```python
from build123d import *

# Parameters (mm, degrees)
CUT_EXTRUDE_1_DEPTH           = 1.2
CUT_EXTRUDE_1_DRAFT           = -30
SKETCH_3_W                    = 3
SKETCH_3_H                    = 12
CUT_EXTRUDE_1_PROFILE_2_DEPTH = 1.2
CUT_EXTRUDE_1_PROFILE_2_DRAFT = -30


with BuildPart() as part:
    # Эскиз1 → Повернуть1 (revolve)
    with BuildSketch(Plane.XY, mode=Mode.PRIVATE) as revolve_1_sk:
        with BuildLine():
            Line((0, 64.100995099), (-26.732050808, 64.100995099))
            Line((-26.732050808, 64.100995099), (-30.196152423, 58.100995099))
            Line((-30.196152423, 58.100995099), (-26.732050808, 58.100995099))
            Line((-26.732050808, 58.100995099), (-25, 61.100995099))
            Line((-25, 61.100995099), (-20, 61.100995099))
            Line((-20, 61.100995099), (-20, 42.100995099))
            Line((-20, 42.100995099), (-19, 41.100995099))
            Line((-19, 41.100995099), (-18, 41.100995099))
            Line((-18, 41.100995099), (-18, 58.100995099))
            ThreePointArc((-18, 58.100995099), (-17.121320344, 60.222315442), (-15, 61.100995099))
            Line((-15, 61.100995099), (0, 61.100995099))
            Line((0, 61.100995099), (0, 64.100995099))
        make_face()
    revolve(revolve_1_sk.sketch.rotate(Axis((0, 61.100995099, 0), (0, 1, 0)), 270), axis=Axis((0, 61.100995099, 0), (0, 1, 0)))


with BuildPart() as cut_extrude_1_tool:
    # Эскиз3 → Вырез-Вытянуть1 (with draft: the straight prism first)
    with BuildSketch(Plane(origin=(0, 64.100995099, 0), x_dir=(1, 0, 0), z_dir=(0, 1, 0))):
        with BuildLine():
            Line((-4.5, 12.196310918), (-4.5, 8.93028555))
            ThreePointArc((-4.5, 8.93028555), (0, -10), (4.5, 8.93028555))
            Line((4.5, 8.93028555), (4.5, 12.196310918))
            ThreePointArc((4.5, 12.196310918), (0, -13), (-4.5, 12.196310918))
        make_face()
    extrude(amount=-CUT_EXTRUDE_1_DEPTH)
    # Вырез-Вытянуть1: the draft: its side faces are tilted about the plane it starts from
    cut_extrude_1_sides = [cut_extrude_1_tool.faces().sort_by_distance(p)[0] for p in [
        (-4.5, 63.500995099, -10.563298234),
        (0, 63.500995099, 10),
        (4.5, 63.500995099, -10.563298234),
        (0, 63.500995099, 13),
    ]]
    draft(cut_extrude_1_sides, Plane(origin=(0, 64.100995099, 0), x_dir=(1, 0, 0), z_dir=(0, 1, 0)), CUT_EXTRUDE_1_DRAFT)


with BuildPart() as part_1:
    add(part.part)

    # Вырез-Вытянуть1: cut by cut_extrude_1_tool
    add(cut_extrude_1_tool.part, mode=Mode.SUBTRACT)


with BuildPart() as cut_extrude_1_profile_2_tool:
    # Эскиз3 → Вырез-Вытянуть1 profile 2 (with draft: the straight prism first)
    with BuildSketch(Plane(origin=(0, 64.100995099, 0), x_dir=(1, 0, 0), z_dir=(0, 1, 0))):
        with Locations((0, 11.509630879)):
            Rectangle(SKETCH_3_W, SKETCH_3_H)
    extrude(amount=-CUT_EXTRUDE_1_PROFILE_2_DEPTH)
    # Вырез-Вытянуть1 profile 2: the draft: its side faces are tilted about the plane it starts from
    cut_extrude_1_profile_2_sides = [cut_extrude_1_profile_2_tool.faces().sort_by_distance(p)[0] for p in [
        (-1.5, 63.500995099, -11.509630879),
        (0, 63.500995099, -5.509630879),
        (1.5, 63.500995099, -11.509630879),
        (0, 63.500995099, -17.509630879),
    ]]
    draft(cut_extrude_1_profile_2_sides, Plane(origin=(0, 64.100995099, 0), x_dir=(1, 0, 0), z_dir=(0, 1, 0)), CUT_EXTRUDE_1_PROFILE_2_DRAFT)


with BuildPart() as part_2:
    add(part_1.part)

    # Вырез-Вытянуть1 profile 2: cut by cut_extrude_1_profile_2_tool
    add(cut_extrude_1_profile_2_tool.part, mode=Mode.SUBTRACT)


solid = part_2.part
```
The model under review builds one solid part; all positions refer to its coordinate system, in mm. A direction names the side the tool comes from. Round coordinates to 2 decimals unless told otherwise and drop trailing zeros. Write each loop counter-clockwise with the first axis right and the second up, starting at its lowest first coordinate (ties: lowest second). Pieces come first, ordered by that corner, then holes. Notation, with made-up numbers: (-2, 38.5) - (8, 38.5) arc R18 ccw to (8, 48.5) - close; hole circle Ø6 at (47, 7.25). An arc over 180 degrees is marked (long way). One line per question, with ' | ' between items.
Item 1: For faces 5 (the face through (17, 41.101, -7)), 6 (the face through (-1, 62.901, 11)), 7 (the face through (-17, 61.101, 11)), list the 3-axis set-ups (+Z, -Z, +X, -X, +Y, -Y) from which the entire face can be reached by the end or side of a thin tool; tool diameter is ignored.
Resolved:
face 5: +Z, -Z, +X, -X, -Y | face 6: +Y | face 7: -Y
Item 2: The part is to be moulded in two halves that separate along Z. For faces 1 (the face through (0, 62.901, -12)), 2 (the face through (24.488, 60.955, 5.438)), 3 (the face through (26.308, 63.726, 5.842)), 4 (the face through (0, 64.101, 0)), say which applies: pulls with the +Z half, pulls with the -Z half, needs draft (parallel to the pull), parting line crosses it, or undercut.
Resolved:
face 1: undercut | face 2: undercut | face 3: parting line crosses it | face 4: needs draft
Item 3: Add section B-B, the plane x = 0. Give the boundary of the cut face in (y, z).
Resolved:
outline: (41.1, -19) - (42.1, -20) - (61.1, -20) - (61.1, -25) - (58.1, -26.73) - (58.1, -30.2) - (64.1, -26.73) - (64.1, -17.51) - (62.9, -16.82) - (62.9, -6.2) - (64.1, -5.51) - (64.1, 10) - (62.9, 10.69) - (62.9, 12.31) - (64.1, 13) - (64.1, 26.73) - (58.1, 30.2) - (58.1, 26.73) - (61.1, 25) - (61.1, 20) - (42.1, 20) - (41.1, 19) - (41.1, 18) - (58.1, 18) arc R3 cw to (61.1, 15) - (61.1, -15) arc R3 cw to (58.1, -18) - (41.1, -18) - close
Item 4: To check wall thickness, follow probe 1 along X at (y, z) = (49, 0); probe 2 along Y at (x, z) = (-5.5, 7); probe 3 along X at (y, z) = (60.5, 13). State the ranges of each line that lie inside material, in increasing order.
Resolved:
probe 1: x = -20 to -18, 18 to 20 | probe 2: y = 61.1 to 64.1 | probe 3: x = -25.71 to -21.76, -15.2 to -10.64, 10.64 to 15.2, 21.76 to 25.71
Item 5: For P1, Ø1, axis at x = 12.5, z = -6, coming from the -Y side; P2, Ø8, axis at x = -21.5, z = 23, coming from the +Y side; P3, Ø12, axis at y = 49, z = 11.5, coming from the -X side; P4, Ø3, axis at y = 55.5, z = -23.5, coming from the +X side, all flat-tipped, find the tip position at first contact; note any pin that passes through.
Resolved:
P1: stops at y = 61.1 | P2: stops at y = 62.8 | P3: stops at x = -19.23 | P4: passes through
Item 6: Add section A-A, the plane z = 0. Give the boundary of the cut face in (x, y), then the cut area to 3 significant figures.
Resolved:
outline: (-30.2, 58.1) - (-26.73, 58.1) - (-25, 61.1) - (-20, 61.1) - (-20, 42.1) - (-19, 41.1) - (-18, 41.1) - (-18, 58.1) arc R3 cw to (-15, 61.1) - (15, 61.1) arc R3 cw to (18, 58.1) - (18, 41.1) - (19, 41.1) - (20, 42.1) - (20, 61.1) - (25, 61.1) - (26.73, 58.1) - (30.2, 58.1) - (26.73, 64.1) - (13, 64.1) - (12.31, 62.9) - (10.69, 62.9) - (10, 64.1) - (-10, 64.1) - (-10.69, 62.9) - (-12.31, 62.9) - (-13, 64.1) - (-26.73, 64.1) - close | area: 264 mm2
Item 7: Add section C-C, the plane y = 55.75. Give the boundary of the cut face in (x, z).
Resolved:
outline: circle Ø40 at (0, 0); hole circle Ø36 at (0, 0)
